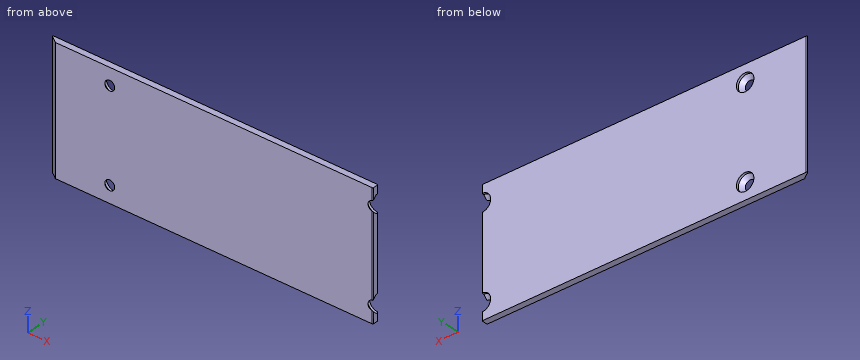
```python
from build123d import *

# Parameters (mm, degrees)
AUFSATZ_LINEAR_START                        = -8.5
AUFSATZ_LINEAR_AUSTRAGEN1_DEPTH             = 41
VERRUNDUNG1_R                               = 0.5
FORMSENKUNG_F_R_M5_SENKSCHRAUBE_MIT_2_COUNT = 2
FORMSENKUNG_F_R_M5_SENKSCHRAUBE_MIT_2_PITCH = 173


with BuildPart() as part:
    # Skizze2 → Aufsatz-Linear austragen1 (new body)
    with BuildSketch(Plane.XY.offset(AUFSATZ_LINEAR_START)):
        with BuildLine():
            Line((9.797958971, 23), (225, 23))
            Line((225, 23), (225, 19))
            Line((225, 19), (17.007351352, 19))
            Line((17.007351352, 19), (16.248076809, 19))
            ThreePointArc((16.248076809, 19), (13.175697134, 21.246199779), (9.797958971, 23))
        make_face()
    extrude(amount=-AUFSATZ_LINEAR_AUSTRAGEN1_DEPTH)

    # Verrundung1
    verrundung1_edges = [part.edges().sort_by_distance(p)[0] for p in [
        (16.248076809, 19, -29),
        (9.797958971, 23, -29),
        (225, 23, -29),
        (225, 19, -29),
    ]]
    fillet(verrundung1_edges, radius=VERRUNDUNG1_R)

    # Skizze6 → Formsenkung für M5 Senkschraube mit Innensechskant1 (revolve, cut)
    with BuildSketch(Plane(origin=(225, 23, -19.5), x_dir=(0, 0, 1), z_dir=(1, 0, 0))):
        Polygon((0, 0), (0, 5.652366702), (2.75, 4), (2.75, 4.485), (5.735, 1.5), (5.735, 0), align=None)
    formsenkung_f_r_m5_senkschraube_mit_inne = revolve(axis=Axis((225, 29.35, -19.5), (0, -1, 0)), mode=Mode.SUBTRACT)

    # Formsenkung f_r M5 Senkschraube mit  2: Formsenkung für M5 Senkschraube mit Innensechskant1 ×2
    with Locations(*[(-i * FORMSENKUNG_F_R_M5_SENKSCHRAUBE_MIT_2_PITCH, 0, 0) for i in range(1, FORMSENKUNG_F_R_M5_SENKSCHRAUBE_MIT_2_COUNT)]):
        add(formsenkung_f_r_m5_senkschraube_mit_inne, mode=Mode.SUBTRACT)

    # Spiegeln2: part across plane


with BuildPart() as part_1:
    add(part.part)
    add(part.part.mirror(Plane.XY.offset(-49.5)))


solid = part_1.part
```
Build history of the part. All positions in model axes, mm. Coordinates: 2 decimals unless noted, no trailing zeros. Write each loop counter-clockwise with the first axis right and the second up, starting at its lowest first coordinate (ties: lowest second). Pieces come first, ordered by that corner, then holes.
1. Band-saw the part on B-B, the plane y = 20.35. Give the cut face in (x, z) (3 decimals).
Answer block:
outline: (14.522, -90.5) - (225, -90.5) - (225, -84.085) arc R4.585 cw to (225, -74.915) - (225, -24.085) arc R4.585 cw to (225, -14.915) - (225, -8.5) - (14.522, -8.5) - close; hole circle Ø9.17 at (52, -79.5); hole circle Ø9.17 at (52, -19.5)
2. Drop flat-ended pins along their axis: pin 1 (1.5 mm diameter, centred on y = 20.5, z = -38, fed in from -X); pin 2 (1 mm diameter, centred on y = 21.5, z = -21.5, fed in from -X); pin 3 (10.5 mm diameter, centred on x = 52, z = -79.5, fed in from +Y) (3 decimals). Give the stop position or say it passes through.
Answer block:
pin 1: stops at x = 13.17
pin 2: stops at x = 11.87
pin 3: stops at y = 21.015
3. Drill centre lines: probe 1 along Z at (x, y) = (52, 21.95) (3 decimals); probe 2 along X at (y, z) = (22.65, -19.5) (3 decimals); probe 3 along X at (y, z) = (21.95, -19.5) (3 decimals). Where is each one in solid material? Low to high.
Answer block:
probe 1: z = -90.5 to -85.235, -73.765 to -25.235, -13.765 to -8.5
probe 2: x = 11.523 to 46.265, 57.735 to 219.265
probe 3: x = 11.967 to 46.265, 57.735 to 219.265
4. Band-saw the part on C-C, the plane x = 52. Give the cut face in (y, z) (3 decimals), and give its area (3 significant figures).
Answer block:
outline: (19, -90.5) - (23, -90.5) - (23, -85.235) - (21.5, -85.235) - (19, -82.735) - close; (19, -76.265) - (21.5, -73.765) - (23, -73.765) - (23, -25.235) - (21.5, -25.235) - (19, -22.735) - close; (19, -16.265) - (21.5, -13.765) - (23, -13.765) - (23, -8.5) - (19, -8.5) - close
area: 249 mm2
5. Band-saw the part on A-A, the plane z = -79.5. Give the cut face in (x, y) (3 decimals), and give its area (3 significant figures).
Answer block:
outline: (11.765, 22.059) arc R25 cw to (16.109, 19.118) arc R0.5 ccw to (16.432, 19) - (48.765, 19) - (46.265, 21.5) - (46.265, 23) - (12, 23) arc R0.5 ccw to start; (55.235, 19) - (221.765, 19) - (219.265, 21.5) - (219.265, 23) - (57.735, 23) - (57.735, 21.5) - close
area: 786 mm2
